Source: CAD feature listing. Evaluate the final solid. Frame: model axes, mm. A direction names the side the tool comes from. Give positions to 0.01 mm unless a question says otherwise; leave off trailing zeros. Write each loop counter-clockwise with the first axis right and the second up, starting at its lowest first coordinate (ties: lowest second). Pieces come first, ordered by that corner, then holes. Notation, with made-up numbers: (16.25, -4) -> (25.25, -4) arc R19 cw to (25.25, 9) -> close; hole circle Ø9 at (-39, 53). An arc over 180 degrees is marked (long way). Answer as a JSON object with one key per item and string values. Group by question number.
Item 1: Access query for faces 1 (the face through (20.21, 0.99, 10.37)), 2 (the face through (-7.551, -11, -3)). Directions: +Z, -Z, +X, -X, +Y, -Y. A direction counts if a zero-diameter tool reaches every point of the face in a straight line with its end or side. Return the directions, or none.
Item 2: Section query D-D on y = -6. Return the cut outline in (x, z), plus the area to 3 significant figures.
Item 3: First-contact query: pin 1 Ø3.5 at (x, z) = (-4.55, -16.28) entering from -Y; pin 2 Ø3.5 at (y, z) = (-20, -3.28) entering from +X. Flat tips, straight axial feed; report the tip coordinate or a pass-through.
Item 4: Section query C-C on x = 16. Return the cut outline in (y, z).
Item 5: Section query B-B on z = -20.5. Return the cut outline in (x, y).
Item 6: Pull-direction query (Y, two-part tool) for faces 3 (the face through (-7.804, -18.986, -4.383)), 4 (the face through (10, 1, 16.723)), 5 (the face through (10, 2, -4)), 6 (the face through (11, 0, -4)); classes: pulls with the +Y half, pulls with the -Y half, needs draft (parallel to the pull), parting line crosses it, or undercut.
Item 7: Ray query, probe 1 along Y at (x, z) = (6.5, -19.5); probe 2 along X at (y, z) = (-1, 5). Return the intervals inside material, ascending. Write a range as from..to.
Item 8: Section query A-A on y = -20. Return the cut outline in (x, z).
from build123d import *

# Parameters (mm, degrees)
SKETCH_1_W        = 40
SKETCH_1_H        = 40
SKETCH_1_R        = 1.4
EXTRUDE_494_DEPTH = 2
SKETCH_2_R        = 1.5
EXTRUDE_1_DEPTH   = 2
CHAMFER_1_SIZE    = 1.5


with BuildPart() as part:
    # Sketch 1 → Extrude 494 (new body)
    with BuildSketch(Plane(origin=(0, 0, 0), x_dir=(1, 0, 0), z_dir=(0, 1, 0))):
        with Locations((10.449336465, 3.276993421)):
            Rectangle(SKETCH_1_W, SKETCH_1_H)
        with Locations(Location((-4.550663535, 16.276993421, 0), (0, 0, 270))):
            Circle(SKETCH_1_R, mode=Mode.SUBTRACT)
        with Locations(Location((21.449336465, 16.276993421, 0), (0, 0, 270))):
            Circle(SKETCH_1_R, mode=Mode.SUBTRACT)
        with Locations(Location((21.449336465, -9.723006579, 0), (0, 0, 270))):
            Circle(SKETCH_1_R, mode=Mode.SUBTRACT)
        with Locations(Location((-4.550663535, -9.723006579, 0), (0, 0, 270))):
            Circle(SKETCH_1_R, mode=Mode.SUBTRACT)
    extrude(amount=EXTRUDE_494_DEPTH)

    # Sketch 2 → Extrude 1 (add)
    with BuildSketch(Plane.ZY.offset(9.550663535)):
        with BuildLine():
            Line((-12.391371699, -24.114378278), (-23.276993421, 0))
            Line((-23.276993421, 0), (16.723006579, 0))
            Line((16.723006579, 0), (5.837384857, -24.114378278))
            ThreePointArc((5.837384857, -24.114378278), (-3.276993421, -30), (-12.391371699, -24.114378278))
        make_face()
        with Locations((-3.276993421, -20)):
            Circle(SKETCH_2_R, mode=Mode.SUBTRACT)
    extrude(amount=-EXTRUDE_1_DEPTH)

    # Chamfer 1
    chamfer_1_edges = [part.edges().sort_by_distance(p)[0] for p in [
        (-9.550663535, -20, -4.776993421),
    ]]
    chamfer(chamfer_1_edges, length=CHAMFER_1_SIZE)


solid = part.part
Worked answers:
{
 "1": {"face 1": "+Y, -Y", "face 2": "+Z, -Z, +X, -Y"},
 "2": {"outline": "(-9.55, -20.57) -> (-7.55, -20.57) -> (-7.55, 14.01) -> (-9.55, 14.01) -> close", "area": "69.2 mm^2"},
 "3": {"pin 1": "y = 0", "pin 2": "x = -7.55"},
 "4": {"outline": "(0, -23.28) -> (2, -23.28) -> (2, 16.72) -> (0, 16.72) -> close"},
 "5": {"outline": "(-9.55, -6.15) -> (-7.55, -6.15) -> (-7.55, 0) -> (30.45, 0) -> (30.45, 2) -> (-9.55, 2) -> close"},
 "6": {"face 3": "undercut", "face 4": "needs draft", "face 5": "pulls with the +Y half", "face 6": "pulls with the -Y half"},
 "7": {"probe 1": "0..2", "probe 2": "-9.55..-7.55"},
 "8": {"outline": "(-9.55, -14.25) -> (-7.55, -14.25) -> (-7.55, -4.78) -> (-8.05, -4.78) -> (-9.55, -6.28) -> close; (-9.55, -0.28) -> (-8.05, -1.78) -> (-7.55, -1.78) -> (-7.55, 7.69) -> (-9.55, 7.69) -> close"}
}
